from build123d import *

# Parameters (mm, degrees)
ESQUISSE1_W             = 19
ESQUISSE1_H             = 39
BOSS_EXTRU_1_DEPTH      = 38
BOSS_EXTRU_2_DEPTH      = 7
BOSS_EXTRU_2_DEPTH_BACK = 46
ESQUISSE2_W             = 19
ESQUISSE2_H             = 2
ESQUISSE3_R             = 2.95
BOSS_EXTRU_3_DEPTH      = 4


with BuildPart() as part:
    # Esquisse1 → Boss.-Extru.1 (new body)
    with BuildSketch(Plane(origin=(0, 0, 0), x_dir=(1, 0, 0), z_dir=(0, 1, 0))):
        with Locations((-9.5, 19.5)):
            Rectangle(ESQUISSE1_W, ESQUISSE1_H)
    extrude(amount=BOSS_EXTRU_1_DEPTH)

    # Esquisse2 → Boss.-Extru.2 (add, two sides: drawn at the far end of the back side and taken through both)
    with BuildSketch(Plane(origin=(0, 0, -39), x_dir=(-1, 0, 0), z_dir=(0, 0, -1)).offset(-BOSS_EXTRU_2_DEPTH_BACK)):
        with Locations((9.5, 26)):
            Rectangle(ESQUISSE2_W, ESQUISSE2_H)
    extrude(amount=BOSS_EXTRU_2_DEPTH + BOSS_EXTRU_2_DEPTH_BACK)

    # Esquisse3 → Boss.-Extru.3 (add)
    with BuildSketch(Plane(origin=(0, 38, 0), x_dir=(1, 0, 0), z_dir=(0, 1, 0))):
        with Locations(Location((-9.5, 29.5, 0), (0, 0, 270))):
            Circle(ESQUISSE3_R)
    extrude(amount=BOSS_EXTRU_3_DEPTH)


solid = part.part
Input: part model. Units: mm. Frame: model coordinates. A direction names the side the tool comes from. Give positions to 0.01 mm unless a question says otherwise; leave off trailing zeros. Loops run counter-clockwise (first coordinate to the right, second up) from the corner with the lowest first, then second, coordinate; pieces in that order, holes last. Notation, with made-up numbers: (17.25, -38) - (70.25, -38) arc R33 cw to (70.25, 1) - close; hole circle Ø1 at (-3, -2). An arc over 180 degrees is marked (long way). Use CSV: the item, a comma, the result in double quotes. Start each with the question number.
Item 1: Section A-A on z = -29.5. Return loops of the section in (x, y).
Item 2: Line query: line 1 (Z direction, x = -3.25, y = 15.5); line 2 (Y direction, x = -12, z = -21.5); line 3 (Y direction, x = -1.5, z = 0.5). Output: solid intervals per line, ascending.
Item 3: Contact query for flat-ended pins moving along their axis: P1, Ø1.5, axis at x = -9.5, z = -40.5, coming from the -Y side; P2, Ø1.5, axis at x = -8, z = -7, coming from the +Y side; P3, Ø7.5, axis at x = -9.5, z = 4, coming from the +Y side. Output: stop coordinate, or through.
Item 4: Reachability of faces 1 (the flat face through (-9, 25, -42)), 2 (the flat face through (-10, 32, 0)), 3 (the flat face through (-9, 25, 4)), 4 (the cylindrical face through (-8.614, 39.972, -26.686)) from +Z, -Z, +X, -X, +Y, -Y: full face, straight path, thin tool, end or side. Return the list, or none.
Item 5: Section C-C on y = 39. Return loops of the section in (x, z), then the cut area to 3 significant figures.
Item 6: Section B-B on x = -9.5. Return loops of the section in (y, z).
Item 7: Section D-D on x = -17.75. Return loops of the section in (y, z), then the cut area to 3 significant figures.
Ans:
1,outline,"(-19, 0) - (0, 0) - (0, 38) - (-6.55, 38) - (-6.55, 42) - (-12.45, 42) - (-12.45, 38) - (-19, 38) - close"
2,line 1,"z = -39 to 0"
2,line 2,"y = 0 to 38"
2,line 3,"y = 25 to 27"
3,P1,"stops at y = 25"
3,P2,"stops at y = 38"
3,P3,"stops at y = 27"
4,face 1,"-Z, +X, -X, -Y"
4,face 2,"+Z, +X, -X, +Y"
4,face 3,"+Z, +X, -X, -Y"
4,face 4,"+Y"
5,outline,"circle Ø5.9 at (-9.5, -29.5)"
5,area,"27.3 mm2"
6,outline,"(0, -39) - (25, -39) - (25, -46) - (27, -46) - (27, -39) - (38, -39) - (38, -32.45) - (42, -32.45) - (42, -26.55) - (38, -26.55) - (38, 0) - (27, 0) - (27, 7) - (25, 7) - (25, 0) - (0, 0) - close"
7,outline,"(0, -39) - (25, -39) - (25, -46) - (27, -46) - (27, -39) - (38, -39) - (38, 0) - (27, 0) - (27, 7) - (25, 7) - (25, 0) - (0, 0) - close"
7,area,"1,510 mm2"
